Work out the finished part from the listing and answer in its coordinate system (mm). Face numbers are marked on the shaded views. Round coordinates to 2 decimals unless told otherwise and drop trailing zeros. Loops run counter-clockwise (first coordinate to the right, second up) from the corner with the lowest first, then second, coordinate; pieces in that order, holes last.
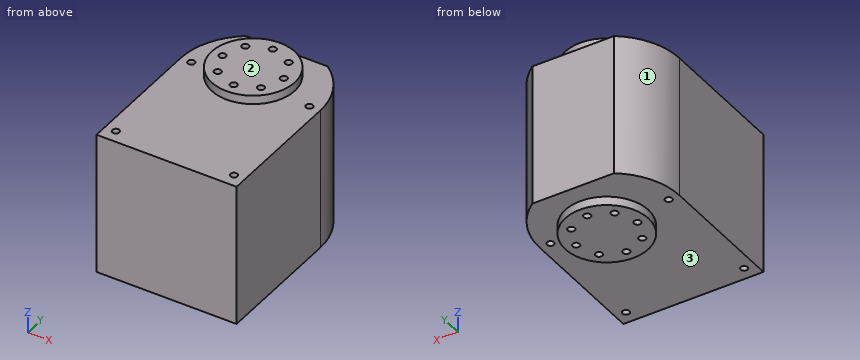
from build123d import *

# Parameters (mm, degrees)
SKETCH_1_R          = 0.8
SKETCH_1_R_2        = 1.5
EXTRUDE_1_DEPTH     = 32.5
SKETCH_2_R          = 4.5
EXTRUDE_2_DEPTH     = 1.5
SKETCH_3_R          = 9.5
EXTRUDE_3_DEPTH     = 2
CUT_EXTRUDE_1_REACH = 50.332
SKETCH_4_R          = 0.8


with BuildPart() as part:
    # Sketch 1 → Extrude 1 (new body)
    with BuildSketch(Plane.XY):
        with BuildLine():
            Line((-9.327379053, 28), (9.327379053, 28))
            ThreePointArc((9.327379053, 28), (14.234431229, 22.306227999), (16, 15))
            Line((16, 15), (16, -15))
            Line((16, -15), (-16, -15))
            Line((-16, -15), (-16, 15))
            ThreePointArc((-16, 15), (-14.234431229, 22.306227999), (-9.327379053, 28))
        make_face()
        with Locations((-13.5, -12)):
            Circle(SKETCH_1_R, mode=Mode.SUBTRACT)
        with Locations((13.5, -12)):
            Circle(SKETCH_1_R, mode=Mode.SUBTRACT)
        with Locations((-13.5, 15)):
            Circle(SKETCH_1_R, mode=Mode.SUBTRACT)
        with Locations((13.5, 15)):
            Circle(SKETCH_1_R, mode=Mode.SUBTRACT)
        with Locations((0, 16)):
            Circle(SKETCH_1_R_2, mode=Mode.SUBTRACT)
    extrude(amount=EXTRUDE_1_DEPTH)

    # Sketch 2 → Extrude 2 (add)
    with BuildSketch(Plane(origin=(0, 0, 0), x_dir=(-1, 0, 0), z_dir=(0, 0, -1))):
        with Locations((0, 16)):
            Circle(SKETCH_2_R)
    extrude_2 = extrude(amount=EXTRUDE_2_DEPTH)

    # Sketch 3 → Extrude 3 (add)
    with BuildSketch(Plane(origin=(0, 0, -1.5), x_dir=(-1, 0, 0), z_dir=(0, 0, -1))):
        with Locations((0, 16)):
            Circle(SKETCH_3_R)
    extrude_3 = extrude(amount=EXTRUDE_3_DEPTH)

    # Sketch 4 → Cut-Extrude 1 (cut, up to next)
    with BuildSketch(Plane(origin=(0, 0, -3.5), x_dir=(-1, 0, 0), z_dir=(0, 0, -1)), mode=Mode.PRIVATE) as cut_extrude_1_sk1:
        with Locations((0, 23)):
            Circle(SKETCH_4_R)
    cut_extrude_1_tool1 = extrude(cut_extrude_1_sk1.sketch, amount=-CUT_EXTRUDE_1_REACH, mode=Mode.PRIVATE) & part.part
    # Sketch 4 → Cut-Extrude 1 (cut, up to next)
    with BuildSketch(Plane(origin=(0, 0, -3.5), x_dir=(-1, 0, 0), z_dir=(0, 0, -1)), mode=Mode.PRIVATE) as cut_extrude_1_sk2:
        with Locations((4.949747468, 20.949747468)):
            Circle(SKETCH_4_R)
    cut_extrude_1_tool2 = extrude(cut_extrude_1_sk2.sketch, amount=-CUT_EXTRUDE_1_REACH, mode=Mode.PRIVATE) & part.part
    # Sketch 4 → Cut-Extrude 1 (cut, up to next)
    with BuildSketch(Plane(origin=(0, 0, -3.5), x_dir=(-1, 0, 0), z_dir=(0, 0, -1)), mode=Mode.PRIVATE) as cut_extrude_1_sk3:
        with Locations((7, 16)):
            Circle(SKETCH_4_R)
    cut_extrude_1_tool3 = extrude(cut_extrude_1_sk3.sketch, amount=-CUT_EXTRUDE_1_REACH, mode=Mode.PRIVATE) & part.part
    # Sketch 4 → Cut-Extrude 1 (cut, up to next)
    with BuildSketch(Plane(origin=(0, 0, -3.5), x_dir=(-1, 0, 0), z_dir=(0, 0, -1)), mode=Mode.PRIVATE) as cut_extrude_1_sk4:
        with Locations((4.949747468, 11.050252532)):
            Circle(SKETCH_4_R)
    cut_extrude_1_tool4 = extrude(cut_extrude_1_sk4.sketch, amount=-CUT_EXTRUDE_1_REACH, mode=Mode.PRIVATE) & part.part
    # Sketch 4 → Cut-Extrude 1 (cut, up to next)
    with BuildSketch(Plane(origin=(0, 0, -3.5), x_dir=(-1, 0, 0), z_dir=(0, 0, -1)), mode=Mode.PRIVATE) as cut_extrude_1_sk5:
        with Locations((0, 9)):
            Circle(SKETCH_4_R)
    cut_extrude_1_tool5 = extrude(cut_extrude_1_sk5.sketch, amount=-CUT_EXTRUDE_1_REACH, mode=Mode.PRIVATE) & part.part
    # Sketch 4 → Cut-Extrude 1 (cut, up to next)
    with BuildSketch(Plane(origin=(0, 0, -3.5), x_dir=(-1, 0, 0), z_dir=(0, 0, -1)), mode=Mode.PRIVATE) as cut_extrude_1_sk6:
        with Locations((-4.949747468, 11.050252532)):
            Circle(SKETCH_4_R)
    cut_extrude_1_tool6 = extrude(cut_extrude_1_sk6.sketch, amount=-CUT_EXTRUDE_1_REACH, mode=Mode.PRIVATE) & part.part
    # Sketch 4 → Cut-Extrude 1 (cut, up to next)
    with BuildSketch(Plane(origin=(0, 0, -3.5), x_dir=(-1, 0, 0), z_dir=(0, 0, -1)), mode=Mode.PRIVATE) as cut_extrude_1_sk7:
        with Locations((-7, 16)):
            Circle(SKETCH_4_R)
    cut_extrude_1_tool7 = extrude(cut_extrude_1_sk7.sketch, amount=-CUT_EXTRUDE_1_REACH, mode=Mode.PRIVATE) & part.part
    # Sketch 4 → Cut-Extrude 1 (cut, up to next)
    with BuildSketch(Plane(origin=(0, 0, -3.5), x_dir=(-1, 0, 0), z_dir=(0, 0, -1)), mode=Mode.PRIVATE) as cut_extrude_1_sk8:
        with Locations((-4.949747468, 20.949747468)):
            Circle(SKETCH_4_R)
    cut_extrude_1_tool8 = extrude(cut_extrude_1_sk8.sketch, amount=-CUT_EXTRUDE_1_REACH, mode=Mode.PRIVATE) & part.part
    cut_extrude_1_1 = cut_extrude_1_tool1.solids().sort_by_distance((0, 23, -3.5))[0]
    add(cut_extrude_1_1, mode=Mode.SUBTRACT)
    cut_extrude_1_2 = cut_extrude_1_tool2.solids().sort_by_distance((-4.949747, 20.949747, -3.5))[0]
    add(cut_extrude_1_2, mode=Mode.SUBTRACT)
    cut_extrude_1_3 = cut_extrude_1_tool3.solids().sort_by_distance((-7, 16, -3.5))[0]
    add(cut_extrude_1_3, mode=Mode.SUBTRACT)
    cut_extrude_1_4 = cut_extrude_1_tool4.solids().sort_by_distance((-4.949747, 11.050253, -3.5))[0]
    add(cut_extrude_1_4, mode=Mode.SUBTRACT)
    cut_extrude_1_5 = cut_extrude_1_tool5.solids().sort_by_distance((0, 9, -3.5))[0]
    add(cut_extrude_1_5, mode=Mode.SUBTRACT)
    cut_extrude_1_6 = cut_extrude_1_tool6.solids().sort_by_distance((4.949747, 11.050253, -3.5))[0]
    add(cut_extrude_1_6, mode=Mode.SUBTRACT)
    cut_extrude_1_7 = cut_extrude_1_tool7.solids().sort_by_distance((7, 16, -3.5))[0]
    add(cut_extrude_1_7, mode=Mode.SUBTRACT)
    cut_extrude_1_8 = cut_extrude_1_tool8.solids().sort_by_distance((4.949747, 20.949747, -3.5))[0]
    add(cut_extrude_1_8, mode=Mode.SUBTRACT)
    cut_extrude_1 = cut_extrude_1_1 + cut_extrude_1_2 + cut_extrude_1_3 + cut_extrude_1_4 + cut_extrude_1_5 + cut_extrude_1_6 + cut_extrude_1_7 + cut_extrude_1_8  # Cut-Extrude 1 as one shape, for the pattern or mirror that repeats it

    # Mirror 1: Extrude 2, Extrude 3, Cut-Extrude 1 across plane
    add(extrude_2.mirror(Plane(origin=(0, 0, 16.25), x_dir=(1, 0, 0), z_dir=(0, 0, -1))))
    add(extrude_3.mirror(Plane(origin=(0, 0, 16.25), x_dir=(1, 0, 0), z_dir=(0, 0, -1))))
    add(cut_extrude_1.mirror(Plane(origin=(0, 0, 16.25), x_dir=(1, 0, 0), z_dir=(0, 0, -1))), mode=Mode.SUBTRACT)


solid = part.part
Item 1: Section C-C, the plane x = 8.5 is taken. Give the vertices of the cut face in (y, z).
Item 2: Section B-B, the plane z = 31.5 is taken. Give the vertices of the cut face in (x, y).
Item 3: Straight lines are drawn through the part: line 1 (Z direction, x = 1, y = 7); line 2 (Y direction, x = 13.5, z = 18); line 3 (Z direction, x = 3, y = 2). For each, find the intervals that lie inside material, in ascending order.
Item 4: Section D-D, the plane x = 0 is taken. State how many separate pieces and enclosed holes the cut face has, plus the area to 3 significant figures.
Item 5: Section A-A, the plane y = -12 is taken. Give the vertices of the cut face in (x, z), plus the area to 3 significant figures.
Item 6: Determine the mould class of the marked faces 1, 2 and 3 for opening direction Z: pulls with the +Z half, pulls with the -Z half, needs draft (parallel to the pull), parting line crosses it, or undercut.
Item 7: Each of these flat-tipped pins is pushed along its axis until it touches: P1, Ø1, axis at x = 4.95, y = 11.05, coming from the -Z side; P2, Ø1.3, axis at x = -4.95, y = 11.05, coming from the +Z side. Where does it stop, or does it pass through?
Answer below:
1. outline: (-15, 0) - (28, 0) - (28, 32.5) - (-15, 32.5) - close; (11.76, -3.5) - (20.24, -3.5) - (20.24, -1.5) - (11.76, -1.5) - close; (11.76, 34) - (20.24, 34) - (20.24, 36) - (11.76, 36) - close
2. outline: (-16, -15) - (16, -15) - (16, 15) arc R16 ccw to (9.33, 28) - (-9.33, 28) arc R16 ccw to (-16, 15) - close; hole circle Ø1.6 at (-13.5, -12); hole circle Ø1.6 at (-13.5, 15); hole circle Ø3 at (0, 16); hole circle Ø1.6 at (13.5, -12); hole circle Ø1.6 at (13.5, 15)
3. line 1: z = -3.5 to -1.5, 0 to 32.5, 34 to 36
3. line 2: y = -15 to -12.8, -11.2 to 14.2, 15.8 to 23.59
3. line 3: z = 0 to 32.5
4. separate pieces: 5
4. enclosed holes: 1
4. area: 1,390 mm2
5. outline: (-16, 0) - (-14.3, 0) - (-14.3, 32.5) - (-16, 32.5) - close; (-12.7, 0) - (12.7, 0) - (12.7, 32.5) - (-12.7, 32.5) - close; (14.3, 0) - (16, 0) - (16, 32.5) - (14.3, 32.5) - close
5. area: 936 mm2
6. face 1: needs draft
6. face 2: pulls with the +Z half
6. face 3: undercut
7. P1: stops at z = 0
7. P2: stops at z = 32.5
